Read the model definition and answer for the solid it produces. Units are mm, in the model's axes. A direction names the side the tool comes from. Give positions to 0.01 mm unless a question says otherwise; leave off trailing zeros. Write each loop counter-clockwise with the first axis right and the second up, starting at its lowest first coordinate (ties: lowest second). Pieces come first, ordered by that corner, then holes. Notation, with made-up numbers: (68, 66) -> (78, 66) arc R17 cw to (78, 90) -> close; hole circle Ø9 at (53, -6). An arc over 180 degrees is marked (long way). Use a Markdown table: item, result.
Autodesk Inventor part; units mm, degrees
ref_plane "YZ Plane" through (0, 0, 0) normal (1, 0, 0) x (0, 1, 0)
ref_plane "XZ Plane" through (0, 0, 0) normal (0, 1, 0) x (-1, 0, 0)
ref_plane "XY Plane" through (0, 0, 0) normal (0, 0, 1) x (1, 0, 0)
sketch "Sketch1" plane through (0, 0, 0) normal (0, 0, 1) x (1, 0, 0)
  line L0 (0, 0) -> (20.066, 0)
  line L1 (20.066, 0) -> (20.066, 88.9)
  line L2 (20.066, 88.9) -> (0, 88.9)
  line L3 (0, 88.9) -> (0, 0)
  circle A0 centre (10.033, 8) radius 2.25
  circle A1 centre (10.033, 23) radius 2.25
  dimension "d0" = 20.066
  dimension "d1" = 88.9
  dimension "d10" = 8
  dimension "d11" = 15
  dimension "d12" = 4.5
  dimension "d13" = 4.5
extrude "Extrusion1" add sketch "Sketch1" along normal blind 3.175
sketch "Sketch2" plane through (0, 0, 3.175) normal (0, 0, 1) x (1, 0, 0)
  line L0 (0, 88.9) -> (0, 0)
  line L1 (20.066, 0) -> (20.066, 88.9)
  line L2 (0, 88.9) -> (20.066, 88.9)
  line L3 (20.066, 88.9) -> (20.066, 76.2)
  line L4 (20.066, 76.2) -> (0, 76.2)
  line L5 (0, 76.2) -> (0, 88.9)
  point P0 (0, 76.2)
  dimension "d4" = 12.7
extrude "Extrusion2" add sketch "Sketch2" along normal blind 38.1
sketch "Sketch3" plane through (0, 0, 0) normal (0, 0, -1) x (-1, 0, 0)
  line L0 (-20.066, 0) -> (-20.066, 88.9)
  line L1 (0, 0) -> (-20.066, 0)
  line L2 (0, 88.9) -> (0, 0)
  line L3 (-20.066, 88.9) -> (0, 88.9)
  line L4 (-20.066, 66.04) -> (0, 66.04)
  line L5 (0, 66.04) -> (0, 0)
  line L6 (0, 0) -> (-20.066, 0)
  line L7 (-20.066, 0) -> (-20.066, 66.04)
  point P0 (0, 66.04)
  dimension "d7" = 22.86
extrude "Extrusion3" add sketch "Sketch3" along normal blind 1.524 contours L0 L4 L2 L1
sketch "Sketch4" plane through (10.033, 23, 0) normal (0, 0, 1) x (1, 0, 0)
  circle A0 centre (0, -15) radius 2.25
  circle A1 centre (0, 0) radius 2.25
  point P0 (-10.033, -23)
extrude "Extrusion4" cut sketch "Sketch4" against normal blind 3.175
sketch "Sketch5" plane through (0, 76.2, 3.175) normal (0, -1, 0) x (1, 0, 0)
  line L0 (20.066, 0) -> (0, 0)
  line L1 (20.066, 0) -> (20.066, 38.1)
  line L2 (0, 38.1) -> (20.066, 38.1)
  line L3 (0, 0) -> (0, 38.1)
  circle A0 centre (10.033, 28.575) radius 2.159
  circle A1 centre (10.033, 9.525) radius 2.159
  point P0 (0, -3.175)
  point P1 (10.033, 38.1)
  dimension "d16" = 4.318
  dimension "d17" = 4.318
  dimension "d18" = 9.525
  dimension "d19" = 9.525
extrude "Extrusion5" cut sketch "Sketch5" against normal through all contours A0 | A1
fillet "Fillet1" radius 3.175 1 edges at (10.033, 76.2, 3.175)
chamfer "Chamfer1" distance 2.286 angle 45 2 edges at (7.874, 76.2, 31.75) (7.874, 76.2, 12.7)
fillet "Fillet2" radius 3.175 1 edges at (10.033, 66.04, 0)
properties part number "Tensioner Mount V1_3DPrint"
Item 1: Each of these flat-tipped pins is pushed along its axis until it touches: P1, Ø3.5, axis at x = 10.033, y = 23, coming from the +Z side; P2, Ø8, axis at x = 17, y = 32, coming from the +Z side (3 decimals); P3, Ø1.5, axis at x = 13.5, y = 67, coming from the -Z side; P4, Ø10, axis at x = 14, z = 26.5, coming from the -Y side. Where does it stop, or does it pass through?
Return value:
| item | result |
|---|---|
| P1 | through |
| P2 | z = 3.175 |
| P3 | z = -1.22 |
| P4 | y = 76.2 |
Item 2: A cutting plane is placed at B-B (z = 31.75). Give the vertices of the cut face in (x, y).
Return value:
| item | result |
|---|---|
| outline | (0, 76.2) -> (5.59, 76.2) -> (7.87, 78.49) -> (7.87, 88.9) -> (0, 88.9) -> close; (12.19, 78.49) -> (14.48, 76.2) -> (20.07, 76.2) -> (20.07, 88.9) -> (12.19, 88.9) -> close |
Item 3: A cutting plane is placed at D-D (y = 80). Give the vertices of the cut face in (x, z) (3 decimals), then the cut area to 3 significant figures.
Return value:
| item | result |
|---|---|
| outline | (0, 0) -> (20.066, 0) -> (20.066, 41.275) -> (0, 41.275) -> close; hole circle Ø4.318 at (10.033, 12.7); hole circle Ø4.318 at (10.033, 31.75) |
| area | 799 mm^2 |
Item 4: For a pull along Y with two mould halves and no side action, classify faces 4 (the face through (10, 37, 3.175)), 5 (the face through (8.375, 6.479, 0.793)), 6 (the face through (10, 88.9, 20)), 7 (the face through (9.893, 75.295, 4.13)) as +Y half, -Y half, draft (parallel to the pull), parting line (faces both ways), or undercut.
Return value:
| item | result |
|---|---|
| face 4 | draft |
| face 5 | undercut |
| face 6 | +Y half |
| face 7 | -Y half |
Item 5: A cutting plane is placed at C-C (x = 15.5). Give the vertices of the cut face in (y, z) (3 decimals), then the cut area to 3 significant figures.
Return value:
| item | result |
|---|---|
| outline | (0, -1.524) -> (66.04, -1.524) arc R3.175 cw to (68.752, 0) -> (88.9, 0) -> (88.9, 41.275) -> (76.2, 41.275) -> (76.2, 6.35) arc R3.175 cw to (73.025, 3.175) -> (0, 3.175) -> close |
| area | 870 mm^2 |
Item 6: Straight lines are drawn through the part: line 1 along Z through (x, y) = (10.25, 84) (3 decimals); line 2 along Z through (x, y) = (8, 62) (3 decimals); line 3 along Y through (x, z) = (13.5, 28.5). For each, find the intervals that lie inside material, in ascending order. Write a range as [from, to].
Return value:
| item | result |
|---|---|
| line 1 | [0, 10.552], [14.848, 29.602], [33.898, 41.275] |
| line 2 | [-1.524, 3.175] |
| line 3 | [76.2, 88.9] |
Item 7: A cutting plane is placed at A-A (y = 8). Give the vertices of the cut face in (x, z) (3 decimals).
Return value:
| item | result |
|---|---|
| outline | (0, -1.524) -> (7.783, -1.524) -> (7.783, 3.175) -> (0, 3.175) -> close; (12.283, -1.524) -> (20.066, -1.524) -> (20.066, 3.175) -> (12.283, 3.175) -> close |
Item 8: A tool of negligible diameter and unlimited length cuts with its end or side. For faces 1 (the face through (10, 79, 0)), 2 (the face through (10, 76.2, 24)), 3 (the face through (10, 83, 41.275)), from which of +Z, -Z, +X, -X, +Y, -Y can it reach the whole face along a straight path? Write none if from no direction.
Return value:
| item | result |
|---|---|
| face 1 | -Z, +X, -X, +Y |
| face 2 | +Z, +X, -X, -Y |
| face 3 | +Z, +X, -X, +Y, -Y |
